Geometry: final body of the model. Coordinates: model frame, mm. Face numbers are marked on the shaded views. A direction names the side the tool comes from. Coordinates: 2 decimals unless noted, no trailing zeros. Loops run counter-clockwise (first coordinate to the right, second up) from the corner with the lowest first, then second, coordinate; pieces in that order, holes last. Notation, with made-up numbers: (58, 66) - (79, 66) arc R15 ccw to (79, 78) - close; hole circle Ø4 at (27.25, 34). An arc over 180 degrees is marked (long way). Put each result on its own line as item: value. Start each with the question number.
1) Section C-C on y = 16.5. Output: boundary loops of the cut face in (x, z).
2) Reachability of the marked faces 5, 6 and 7 from +Z, -Z, +X, -X, +Y, -Y: full face, straight path, thin tool, end or side. Return the list, or none.
3) Section B-B on x = 45. Output: boundary loops of the cut face in (y, z), and give its area (3 significant figures).
4) Section A-A on z = -3. Output: boundary loops of the cut face in (x, y), and give its area (3 significant figures).
5) Draft query along X for the marked faces 1, 2, 3 and 4. Return one class per face: +X half, -X half, draft (parallel to the pull), parting line (faces both ways), or undercut.
6) Contact query for flat-ended pins moving along their axis: pin 1 Ø1.5 at (x, z) = (28, -5) entering from +Y; pin 2 Ø6 at (y, z) = (16, 2.5) entering from -X; pin 3 Ø2 at (y, z) = (30, -21) entering from +X. Output: stop coordinate, or through.
7) Section D-D on x = 37. Output: boundary loops of the cut face in (y, z), and give its area (3 significant figures).
8) Material intervals for line 1 along X through (y, z) = (4, 14); line 2 along X through (y, z) = (22, 0); line 3 along Y through (x, z) = (4, 14), sorted ascending. Write a range as from..to.
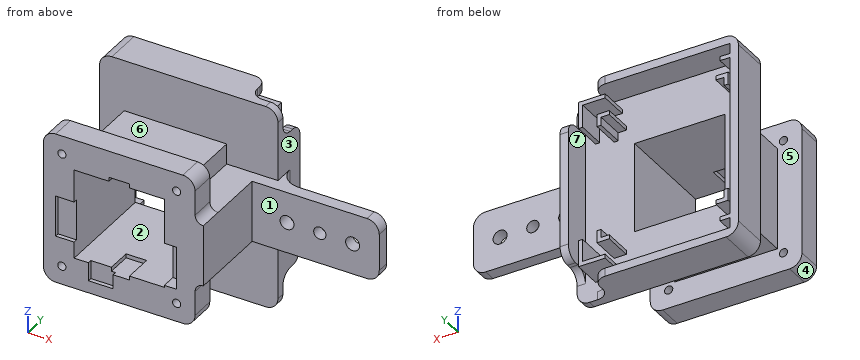
```python
from build123d import *

# Parameters (mm, degrees)
SKETCH_2_W            = 37
SKETCH_2_H            = 37
EXTRUDE_1_DEPTH       = 23
SKETCH_3_W            = 22
SKETCH_3_H            = 22
CUT_EXTRUDE_1_DEPTH   = 23
SKETCH_19_OUTSIDE_W   = 50.432
SKETCH_19_OUTSIDE_H   = 50.432
SKETCH_19_OUTSIDE_W_2 = 25
SKETCH_19_OUTSIDE_H_2 = 25
CUT_EXTRUDE_17_DEPTH  = 17
SKETCH_4_W            = 50
SKETCH_4_H            = 50
EXTRUDE_2_DEPTH       = 9
SKETCH_5_W            = 46
SKETCH_5_H            = 46
CUT_EXTRUDE_3_DEPTH   = 7
SKETCH_12_W           = 8
SKETCH_12_H           = 8
CUT_EXTRUDE_14_DEPTH  = 14
SKETCH_6_W            = 22
SKETCH_6_H            = 22
CUT_EXTRUDE_4_DEPTH   = 2
SKETCH_11_R           = 1
CUT_EXTRUDE_7_DEPTH   = 8
SKETCH_13_W           = 41
SKETCH_13_H           = 41
SKETCH_13_W_2         = 39
SKETCH_13_H_2         = 39
EXTRUDE_3_DEPTH       = 7
SKETCH_17_W           = 32
SKETCH_17_H           = 32
SKETCH_17_W_2         = 30
SKETCH_17_H_2         = 30
EXTRUDE_4_DEPTH       = 7
SKETCH_15_W           = 28
SKETCH_15_H           = 1
SKETCH_15_W_2         = 1
SKETCH_15_H_2         = 28
CUT_EXTRUDE_15_DEPTH  = 7
SKETCH_18_W           = 1
SKETCH_18_H           = 26
SKETCH_18_W_2         = 26
SKETCH_18_H_2         = 1
CUT_EXTRUDE_16_DEPTH  = 7
SKETCH_20_W           = 3
SKETCH_20_H           = 10.5
CUT_EXTRUDE_18_DEPTH  = 3.5
SKETCH_21_W           = 4.5
SKETCH_21_H           = 10
CUT_EXTRUDE_19_DEPTH  = 1
SKETCH_22_W           = 5
SKETCH_22_H           = 1
CUT_EXTRUDE_21_DEPTH  = 7
SKETCH_24_W           = 6
SKETCH_24_H           = 4.5
CUT_EXTRUDE_22_DEPTH  = 1
SKETCH_25_W           = 6
SKETCH_25_H           = 15
EXTRUDE_5_DEPTH       = 17
SKETCH_26_W           = 15
SKETCH_26_H           = 3
EXTRUDE_6_DEPTH       = 33
SKETCH_28_W           = 6.5
SKETCH_28_H           = 50
CUT_EXTRUDE_27_DEPTH  = 13
SKETCH_32_W           = 2
SKETCH_32_H           = 50
EXTRUDE_9_DEPTH       = 9
FILLET_5_R            = 3
FILLET_6_R            = 3
FILLET_7_R            = 3
FILLET_8_R            = 3
FILLET_9_R            = 3
FILLET_10_R           = 3
FILLET_11_R           = 3
FILLET_12_R           = 3
FILLET_13_R           = 3
FILLET_14_R           = 3
FILLET_15_R           = 3
FILLET_16_R           = 3
FILLET_17_R           = 5
FILLET_19_R           = 3
FILLET_20_R           = 3
FILLET_21_R           = 3
FILLET_22_R           = 3
SKETCH_34_W           = 15
SKETCH_34_H           = 20
EXTRUDE_10_DEPTH      = 2
SKETCH_33_R           = 1.7
SKETCH_33_R_2         = 1.5
CUT_EXTRUDE_28_DEPTH  = 7
FILLET_23_R           = 3
FILLET_24_R           = 3
FILLET_25_R           = 2
FILLET_26_R           = 2


with BuildPart() as part:
    # 草图2 → 凸台-拉伸1 (new body)
    with BuildSketch(Plane(origin=(0, 0, 0), x_dir=(1, 0, 0), z_dir=(0, 1, 0))):
        Rectangle(SKETCH_2_W, SKETCH_2_H)
    extrude(amount=EXTRUDE_1_DEPTH)

    # 草图3 → 切除-拉伸1 (cut)
    with BuildSketch(Plane.XZ):
        Rectangle(SKETCH_3_W, SKETCH_3_H)
    extrude(amount=-CUT_EXTRUDE_1_DEPTH, mode=Mode.SUBTRACT)

    # 草图19 outside → 切除-拉伸17 (cut)
    with BuildSketch(Plane(origin=(0, 6, 0), x_dir=(-1, 0, 0), z_dir=(0, -1, 0))):
        Rectangle(SKETCH_19_OUTSIDE_W, SKETCH_19_OUTSIDE_H)
        Rectangle(SKETCH_19_OUTSIDE_W_2, SKETCH_19_OUTSIDE_H_2, mode=Mode.SUBTRACT)
    extrude(amount=-CUT_EXTRUDE_17_DEPTH, mode=Mode.SUBTRACT)

    # 草图4 → 凸台-拉伸2 (add)
    with BuildSketch(Plane(origin=(0, 23, 0), x_dir=(1, 0, 0), z_dir=(0, 1, 0))):
        Rectangle(SKETCH_4_W, SKETCH_4_H)
    extrude(amount=EXTRUDE_2_DEPTH)

    # 草图5 → 切除-拉伸3 (cut)
    with BuildSketch(Plane(origin=(0, 32, 0), x_dir=(1, 0, 0), z_dir=(0, 1, 0))):
        Rectangle(SKETCH_5_W, SKETCH_5_H)
    extrude(amount=-CUT_EXTRUDE_3_DEPTH, mode=Mode.SUBTRACT)

    # 草图12 → 切除-拉伸14 (cut)
    with BuildSketch(Plane(origin=(0, 25, 0), x_dir=(1, 0, 0), z_dir=(0, 1, 0))):
        with Locations((-21, -21)):
            Rectangle(SKETCH_12_W, SKETCH_12_H)
        with Locations((-21, 21)):
            Rectangle(SKETCH_12_W, SKETCH_12_H)
        with Locations((21, 21)):
            Rectangle(SKETCH_12_W, SKETCH_12_H)
        with Locations((21, -21)):
            Rectangle(SKETCH_12_W, SKETCH_12_H)
    extrude(amount=CUT_EXTRUDE_14_DEPTH, mode=Mode.SUBTRACT)

    # 草图6 → 切除-拉伸4 (cut)
    with BuildSketch(Plane(origin=(0, 25, 0), x_dir=(1, 0, 0), z_dir=(0, 1, 0))):
        Rectangle(SKETCH_6_W, SKETCH_6_H)
    extrude(amount=-CUT_EXTRUDE_4_DEPTH, mode=Mode.SUBTRACT)

    # 草图11 → 切除-拉伸7 (cut)
    with BuildSketch(Plane.XZ):
        with Locations(Location((14, 14, 0), (0, 0, 270))):
            Circle(SKETCH_11_R)
        with Locations(Location((14, -14, 0), (0, 0, 270))):
            Circle(SKETCH_11_R)
        with Locations(Location((-14, -14, 0), (0, 0, 270))):
            Circle(SKETCH_11_R)
        with Locations(Location((-14, 14, 0), (0, 0, 270))):
            Circle(SKETCH_11_R)
    extrude(amount=-CUT_EXTRUDE_7_DEPTH, mode=Mode.SUBTRACT)

    # 草图13 → 凸台-拉伸3 (add)
    with BuildSketch(Plane(origin=(0, 25, 0), x_dir=(1, 0, 0), z_dir=(0, 1, 0))):
        Rectangle(SKETCH_13_W, SKETCH_13_H)
        Rectangle(SKETCH_13_W_2, SKETCH_13_H_2, mode=Mode.SUBTRACT)
    extrude(amount=EXTRUDE_3_DEPTH)

    # 草图17 → 凸台-拉伸4 (add)
    with BuildSketch(Plane(origin=(0, 25, 0), x_dir=(1, 0, 0), z_dir=(0, 1, 0))):
        Rectangle(SKETCH_17_W, SKETCH_17_H)
        Rectangle(SKETCH_17_W_2, SKETCH_17_H_2, mode=Mode.SUBTRACT)
    extrude(amount=EXTRUDE_4_DEPTH)

    # 草图15 → 切除-拉伸15 (cut)
    with BuildSketch(Plane(origin=(0, 25, 0), x_dir=(1, 0, 0), z_dir=(0, 1, 0))):
        with Locations((0, -20)):
            Rectangle(SKETCH_15_W, SKETCH_15_H)
        with Locations((20, 0)):
            Rectangle(SKETCH_15_W_2, SKETCH_15_H_2)
        with Locations((-20, 0)):
            Rectangle(SKETCH_15_W_2, SKETCH_15_H_2)
        with Locations((0, 20)):
            Rectangle(SKETCH_15_W, SKETCH_15_H)
    extrude(amount=CUT_EXTRUDE_15_DEPTH, mode=Mode.SUBTRACT)

    # 草图18 → 切除-拉伸16 (cut)
    with BuildSketch(Plane(origin=(0, 25, 0), x_dir=(1, 0, 0), z_dir=(0, 1, 0))):
        with Locations((15.5, 0)):
            Rectangle(SKETCH_18_W, SKETCH_18_H)
        with Locations((0, -15.5)):
            Rectangle(SKETCH_18_W_2, SKETCH_18_H_2)
        with Locations((-15.5, 0)):
            Rectangle(SKETCH_18_W, SKETCH_18_H)
        with Locations((0, 15.5)):
            Rectangle(SKETCH_18_W_2, SKETCH_18_H_2)
    extrude(amount=CUT_EXTRUDE_16_DEPTH, mode=Mode.SUBTRACT)

    # 草图20 → 切除-拉伸18 (cut)
    with BuildSketch(Plane.XZ):
        with Locations((12.5, -5.25)):
            Rectangle(SKETCH_20_W, SKETCH_20_H)
    extrude(amount=-CUT_EXTRUDE_18_DEPTH, mode=Mode.SUBTRACT)

    # 草图21 → 切除-拉伸19 (cut)
    with BuildSketch(Plane.XZ):
        with Locations((-13.25, -2)):
            Rectangle(SKETCH_21_W, SKETCH_21_H)
    extrude(amount=-CUT_EXTRUDE_19_DEPTH, mode=Mode.SUBTRACT)

    # 草图22 → 切除-拉伸21 (cut)
    with BuildSketch(Plane.XZ):
        with Locations((0, -11.5)):
            Rectangle(SKETCH_22_W, SKETCH_22_H)
        with Locations((0, 11.5)):
            Rectangle(SKETCH_22_W, SKETCH_22_H)
    extrude(amount=-CUT_EXTRUDE_21_DEPTH, mode=Mode.SUBTRACT)

    # 草图24 → 切除-拉伸22 (cut)
    with BuildSketch(Plane.XZ):
        with Locations((-4.5, -13.25)):
            Rectangle(SKETCH_24_W, SKETCH_24_H)
    extrude(amount=-CUT_EXTRUDE_22_DEPTH, mode=Mode.SUBTRACT)

    # 草图25 → 凸台-拉伸5 (add)
    with BuildSketch(Plane(origin=(0, 6, 0), x_dir=(1, 0, 0), z_dir=(0, 1, 0))):
        with Locations((15.5, 0)):
            Rectangle(SKETCH_25_W, SKETCH_25_H)
    extrude(amount=EXTRUDE_5_DEPTH)

    # 草图26 → 凸台-拉伸6 (add)
    with BuildSketch(Plane(origin=(18.5, 0, 0), x_dir=(0, 0, -1), z_dir=(1, 0, 0))):
        with Locations((0, 21.5)):
            Rectangle(SKETCH_26_W, SKETCH_26_H)
    extrude(amount=EXTRUDE_6_DEPTH)

    # 草图28 → 切除-拉伸27 (cut)
    with BuildSketch(Plane.XZ.offset(-23)):
        with Locations((-21.75, 0)):
            Rectangle(SKETCH_28_W, SKETCH_28_H)
    extrude(amount=-CUT_EXTRUDE_27_DEPTH, mode=Mode.SUBTRACT)

    # 草图32 → 凸台-拉伸9 (add)
    with BuildSketch(Plane.XZ.offset(-23)):
        with Locations((-17.5, 0)):
            Rectangle(SKETCH_32_W, SKETCH_32_H)
    extrude(amount=-EXTRUDE_9_DEPTH)

    # 圆角5
    fillet_5_edges = [part.edges().sort_by_distance(p)[0] for p in [
        (25, 24, -25),
    ]]
    fillet(fillet_5_edges, radius=FILLET_5_R)

    # 圆角6
    fillet_6_edges = [part.edges().sort_by_distance(p)[0] for p in [
        (25, 24, 25),
    ]]
    fillet(fillet_6_edges, radius=FILLET_6_R)

    # 圆角7
    fillet_7_edges = [part.edges().sort_by_distance(p)[0] for p in [
        (-18.5, 27.5, -25),
    ]]
    fillet(fillet_7_edges, radius=FILLET_7_R)

    # 圆角8
    fillet_8_edges = [part.edges().sort_by_distance(p)[0] for p in [
        (-18.5, 27.5, 25),
    ]]
    fillet(fillet_8_edges, radius=FILLET_8_R)

    # 圆角9
    fillet_9_edges = [part.edges().sort_by_distance(p)[0] for p in [
        (17, 32, -24),
    ]]
    fillet(fillet_9_edges, radius=FILLET_9_R)

    # 圆角10
    fillet_10_edges = [part.edges().sort_by_distance(p)[0] for p in [
        (17, 25, -24),
    ]]
    fillet(fillet_10_edges, radius=FILLET_10_R)

    # 圆角11
    fillet_11_edges = [part.edges().sort_by_distance(p)[0] for p in [
        (24, 32, -17),
    ]]
    fillet(fillet_11_edges, radius=FILLET_11_R)

    # 圆角12
    fillet_12_edges = [part.edges().sort_by_distance(p)[0] for p in [
        (24, 25, -17),
    ]]
    fillet(fillet_12_edges, radius=FILLET_12_R)

    # 圆角13
    fillet_13_edges = [part.edges().sort_by_distance(p)[0] for p in [
        (17, 32, 24),
    ]]
    fillet(fillet_13_edges, radius=FILLET_13_R)

    # 圆角14
    fillet_14_edges = [part.edges().sort_by_distance(p)[0] for p in [
        (17, 25, 24),
    ]]
    fillet(fillet_14_edges, radius=FILLET_14_R)

    # 圆角15
    fillet_15_edges = [part.edges().sort_by_distance(p)[0] for p in [
        (24, 32, 17),
    ]]
    fillet(fillet_15_edges, radius=FILLET_15_R)

    # 圆角16
    fillet_16_edges = [part.edges().sort_by_distance(p)[0] for p in [
        (24, 25, 17),
    ]]
    fillet(fillet_16_edges, radius=FILLET_16_R)

    # 圆角17
    fillet_17_edges = [part.edges().sort_by_distance(p)[0] for p in [
        (25, 23, 0),
    ]]
    fillet(fillet_17_edges, radius=FILLET_17_R)

    # 圆角19
    fillet_19_edges = [part.edges().sort_by_distance(p)[0] for p in [
        (-18.5, 3, -18.5),
    ]]
    fillet(fillet_19_edges, radius=FILLET_19_R)

    # 圆角20
    fillet_20_edges = [part.edges().sort_by_distance(p)[0] for p in [
        (-18.5, 3, 18.5),
    ]]
    fillet(fillet_20_edges, radius=FILLET_20_R)

    # 圆角21
    fillet_21_edges = [part.edges().sort_by_distance(p)[0] for p in [
        (18.5, 3, 18.5),
    ]]
    fillet(fillet_21_edges, radius=FILLET_21_R)

    # 圆角22
    fillet_22_edges = [part.edges().sort_by_distance(p)[0] for p in [
        (18.5, 3, -18.5),
    ]]
    fillet(fillet_22_edges, radius=FILLET_22_R)

    # 草图34 → 凸台-拉伸10 (add)
    with BuildSketch(Plane(origin=(18.5, 0, 0), x_dir=(0, 0, -1), z_dir=(1, 0, 0))):
        with Locations((0, 10)):
            Rectangle(SKETCH_34_W, SKETCH_34_H)
    extrude(amount=EXTRUDE_10_DEPTH)

    # 草图33 → 切除-拉伸28 (cut)
    with BuildSketch(Plane.XZ.offset(-20)):
        with Locations(Location((29, 0, 0), (0, 0, 270))):
            Circle(SKETCH_33_R)
        with Locations(Location((37, 0, 0), (0, 0, 270))):
            Circle(SKETCH_33_R_2)
        with Locations(Location((45, 0, 0), (0, 0, 270))):
            Circle(SKETCH_33_R)
    extrude(amount=-CUT_EXTRUDE_28_DEPTH, mode=Mode.SUBTRACT)

    # 圆角23
    fillet_23_edges = [part.edges().sort_by_distance(p)[0] for p in [
        (51.5, 21.5, 7.5),
    ]]
    fillet(fillet_23_edges, radius=FILLET_23_R)

    # 圆角24
    fillet_24_edges = [part.edges().sort_by_distance(p)[0] for p in [
        (51.5, 21.5, -7.5),
    ]]
    fillet(fillet_24_edges, radius=FILLET_24_R)

    # 圆角25
    fillet_25_edges = [part.edges().sort_by_distance(p)[0] for p in [
        (18.5, 3, 7.5),
    ]]
    fillet(fillet_25_edges, radius=FILLET_25_R - 0.0001)  # a hair under: the kernel refuses the full size

    # 圆角26
    fillet_26_edges = [part.edges().sort_by_distance(p)[0] for p in [
        (18.5, 3, -7.5),
    ]]
    fillet(fillet_26_edges, radius=FILLET_26_R - 0.0001)  # a hair under: the kernel refuses the full size


solid = part.part
```
Answer block:
1. outline: (-12.5, -12.5) - (12.5, -12.5) - (12.5, -7.5) - (20.5, -7.5) - (20.5, 7.5) - (12.5, 7.5) - (12.5, 12.5) - (-12.5, 12.5) - close; hole (-11, -11) - (11, -11) - (11, 11) - (-11, 11) - close
2. face 5: none
2. face 6: +Z, +X, -X
2. face 7: +Z, -Z, +Y
3. outline: (20, -7.5) - (23, -7.5) - (23, -1.7) - (20, -1.7) - close; (20, 1.7) - (23, 1.7) - (23, 7.5) - (20, 7.5) - close
3. area: 34.8 mm²
4. outline: (-18.5, 0) - (-15.5, 0) - (-15.5, 1) - (-11, 1) - (-11, 25) - (-16.5, 25) - (-16.5, 32) - (-18.5, 32) - (-18.5, 23) - (-12.5, 23) - (-12.5, 6) - (-18.5, 6) - close; (11, 3.5) - (14, 3.5) - (14, 0) - (20.5, 0) - (20.5, 20) - (51.5, 20) - (51.5, 23) - (30, 23) arc R5 cw to (25, 28) - (25, 32) - (23, 32) - (23, 25) - (11, 25) - close
4. area: 443 mm²
5. face 1: draft
5. face 2: undercut
5. face 3: +X half
5. face 4: -X half
6. pin 1: stops at y = 23.82
6. pin 2: stops at x = -12.5
6. pin 3: stops at x = 20.5
7. outline: (20, -7.5) - (23, -7.5) - (23, -1.5) - (20, -1.5) - close; (20, 1.5) - (23, 1.5) - (23, 7.5) - (20, 7.5) - close
7. area: 36.0 mm²
8. line 1: x = -18.5..-15, -13..13, 15..18.5
8. line 2: x = -12.5..-11, 11..27.3, 30.7..35.5, 38.5..43.3, 46.7..51.5
8. line 3: y = 0..6, 23..25
